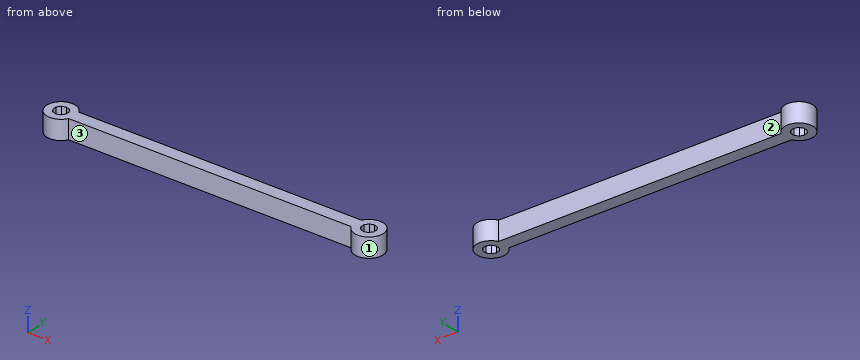
```python
from build123d import *

# Parameters (mm, degrees)
F1_DEPTH = 5


with BuildPart() as f1:
    # F0 (on Top) → F1 (new body)
    with BuildSketch(Plane.XY):
        with BuildLine():
            Line((36.713665, 1.7), (-36.713665, 1.7))
            ThreePointArc((-36.713665, 1.7), (-43.7, 0), (-36.713665, -1.7))
            Line((-36.713665, -1.7), (36.713665, -1.7))
            ThreePointArc((36.713665, -1.7), (43.7, 0), (36.713665, 1.7))
        make_face()
        Polygon((-41.050658, -1.446106), (-41.7, -0.552363), (-41.7, 0.552363), (-41.050658, 1.446106), (-40, 1.787486), (-38.949342, 1.446106), (-38.3, 0.552363), (-38.3, -0.552363), (-38.949342, -1.446106), (-40, -1.787486), align=None, mode=Mode.SUBTRACT)
        Polygon((41.050658, 1.446106), (41.7, 0.552363), (41.7, -0.552363), (41.050658, -1.446106), (40, -1.787486), (38.949342, -1.446106), (38.3, -0.552363), (38.3, 0.552363), (38.949342, 1.446106), (40, 1.787486), align=None, mode=Mode.SUBTRACT)
    extrude(amount=F1_DEPTH)


solid = f1.part
```
Verification items for the finished model (mm, model axes). Face numbers are marked on the shaded views. A direction names the side the tool comes from. Round coordinates to 2 decimals unless told otherwise and drop trailing zeros. Write each loop counter-clockwise with the first axis right and the second up, starting at its lowest first coordinate (ties: lowest second). Pieces come first, ordered by that corner, then holes.
1. Section check C-C on x = 12. Enter the section's corners in (y, z), plus the area to 3 significant figures.
2. Scan lines: L1, parallel to X at y = 0.25, z = 2.8; L2, parallel to Y at x = -40, z = 1.1; L3, parallel to X at y = 1, z = 4.1. Record each from-to range of solid material in increasing order.
3. Access from +Z, -Z, +X, -X, +Y, -Y to the whole of each face (thin tool, end or side, straight path). Record for the marked faces 1, 2 and 3.
4. Section check A-A on z = 2.8. Enter the section's corners in (x, y).
5. Gauge pin test, flat ends, axial feed: P1, Ø3, axis at x = 13.5, z = 0.5, coming from the -Y side; P2, Ø1, axis at y = -2.5, z = 1, coming from the -X side. Record the tip position at first contact, or that the pin passes through.
6. Section check B-B on y = 2.75. Enter the section's corners in (x, z), plus the area to 3 significant figures.
Answer:
1. outline: (-1.7, 0) - (1.7, 0) - (1.7, 5) - (-1.7, 5) - close
1. area: 17.0 mm2
2. L1: x = -43.69 to -41.7, -38.3 to 38.3, 41.7 to 43.69
2. L2: y = -3.7 to -1.79, 1.79 to 3.7
2. L3: x = -43.56 to -41.37, -38.63 to 38.63, 41.37 to 43.56
3. face 1: +Z, -Z
3. face 2: +Z, -Z, +Y
3. face 3: +Z, -Z, -Y
4. outline: (-36.71, -1.7) - (36.71, -1.7) arc R3.7 ccw (long way) to (36.71, 1.7) - (-36.71, 1.7) arc R3.7 ccw (long way) to start; hole (-41.7, -0.55) - (-41.05, -1.45) - (-40, -1.79) - (-38.95, -1.45) - (-38.3, -0.55) - (-38.3, 0.55) - (-38.95, 1.45) - (-40, 1.79) - (-41.05, 1.45) - (-41.7, 0.55) - close; hole (38.3, -0.55) - (38.95, -1.45) - (40, -1.79) - (41.05, -1.45) - (41.7, -0.55) - (41.7, 0.55) - (41.05, 1.45) - (40, 1.79) - (38.95, 1.45) - (38.3, 0.55) - close
5. P1: stops at y = -1.7
5. P2: stops at x = -43.11
6. outline: (-42.48, 0) - (-37.52, 0) - (-37.52, 5) - (-42.48, 5) - close; (37.52, 0) - (42.48, 0) - (42.48, 5) - (37.52, 5) - close
6. area: 49.5 mm2
